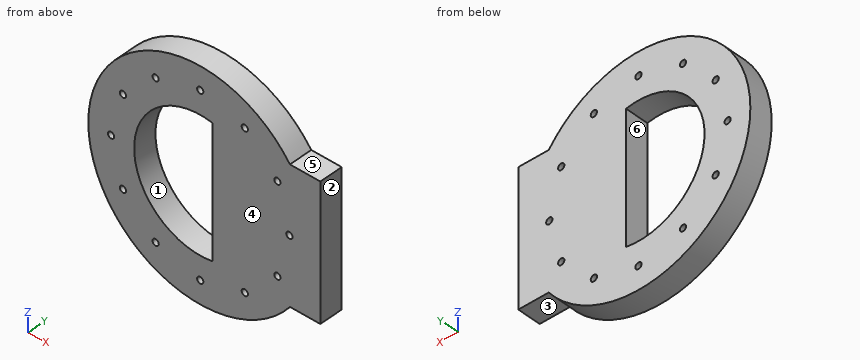
```python
from build123d import *

# Parameters (mm, degrees)
SKETCH1_R           = 127.508
SKETCH1_R_2         = 75.311
SKETCH1_R_3         = 3.5687
BOSS_EXTRUDE1_DEPTH = 26.67
BOSS_EXTRUDE2_DEPTH = 26.67


with BuildPart() as part:
    # Sketch1 → Boss-Extrude1 (new body)
    with BuildSketch(Plane(origin=(0, 0, 0), x_dir=(1, 0, 0), z_dir=(0, 1, 0))):
        Circle(SKETCH1_R)
        Circle(SKETCH1_R_2, mode=Mode.SUBTRACT)
        with Locations((0, 101.6)):
            Circle(SKETCH1_R_3, mode=Mode.SUBTRACT)
        with Locations((50.8, 87.988181024)):
            Circle(SKETCH1_R_3, mode=Mode.SUBTRACT)
        with Locations((87.988181025, 50.8)):
            Circle(SKETCH1_R_3, mode=Mode.SUBTRACT)
        with Locations((101.6, 0)):
            Circle(SKETCH1_R_3, mode=Mode.SUBTRACT)
        with Locations((87.988181025, -50.8)):
            Circle(SKETCH1_R_3, mode=Mode.SUBTRACT)
        with Locations((50.8, -87.988181024)):
            Circle(SKETCH1_R_3, mode=Mode.SUBTRACT)
        with Locations((0, -101.6)):
            Circle(SKETCH1_R_3, mode=Mode.SUBTRACT)
        with Locations((-50.8, -87.988181025)):
            Circle(SKETCH1_R_3, mode=Mode.SUBTRACT)
        with Locations((-87.988181024, -50.8)):
            Circle(SKETCH1_R_3, mode=Mode.SUBTRACT)
        with Locations((-101.6, 0)):
            Circle(SKETCH1_R_3, mode=Mode.SUBTRACT)
        with Locations((-87.988181024, 50.8)):
            Circle(SKETCH1_R_3, mode=Mode.SUBTRACT)
        with Locations((-50.8, 87.988181024)):
            Circle(SKETCH1_R_3, mode=Mode.SUBTRACT)
    extrude(amount=BOSS_EXTRUDE1_DEPTH)

    # Sketch2 → Boss-Extrude2 (add, through all)
    with BuildSketch(Plane(origin=(0, 26.67, 0), x_dir=(1, 0, 0), z_dir=(0, 1, 0))):
        with BuildLine():
            Line((14.224, 73.955557905), (14.224, -73.955557905))
            ThreePointArc((14.224, -73.955557905), (75.311, 0), (14.224, 73.955557905))
        make_face()
        with BuildLine():
            Line((136.906, 76.2), (136.906, -76.2))
            Line((136.906, -76.2), (102.23429006, -76.2))
            ThreePointArc((102.23429006, -76.2), (127.508, 0), (102.23429006, 76.2))
            Line((102.23429006, 76.2), (136.906, 76.2))
        make_face()
    extrude(amount=-BOSS_EXTRUDE2_DEPTH)


solid = part.part
```
Model file for the job. Use its own axes, mm. Face numbers are marked on the shaded views. A direction names the side the tool comes from. Give positions to 0.01 mm unless a question says otherwise; leave off trailing zeros. Loops run counter-clockwise (first coordinate to the right, second up) from the corner with the lowest first, then second, coordinate; pieces in that order, holes last. Notation, with made-up numbers: M 11.25,16.5 L 26.25,16.5 A21 ccw 26.25,29.5 Z; hole C -11,-15 d10. An arc over 180 degrees is marked long. Use one line per item in the form item = value.
Item 1: Two-plate mould, pull along Z, no slides. Class the marked faces 1, 2 and 3: released by +Z, released by -Z, zero draft, split by the parting line, or undercut.
Filled in:
face_1 = undercut
face_2 = zero draft
face_3 = released by -Z
Item 2: Slice it at B-B on z = 68. List the corners of the cut face in (x, y).
Filled in:
outline = M -107.86,0 L -32.37,0 L -32.37,26.67 L -107.86,26.67 Z; M 14.22,0 L 136.91,0 L 136.91,26.67 L 14.22,26.67 Z
Item 3: Slice it at D-D on x = -101.6. List the corners of the cut face in (y, z), and give its area (3 significant figures).
Filled in:
outline = M 0,-77.04 L 26.67,-77.04 L 26.67,-3.57 L 0,-3.57 Z; M 0,3.57 L 26.67,3.57 L 26.67,77.04 L 0,77.04 Z
area = 3,920 mm^2
Item 4: Slice it at C-C on y = 15.5. Give the number of separate pieces and of enclosed holes in the cut face, and give its area (3 significant figures).
Filled in:
separate_pieces = 1
enclosed_holes = 13
area = 42,200 mm^2
Item 5: Drill centre lines: L1, parallel to Z at x = -53.5, y = 4.75; L2, parallel to X at y = 3.5, z = -49.5; L3, parallel to Z at x = 50, y = 23. Where is each one in solid material? Low to high.
Filled in:
L1 = -115.74 to -90.32, -85.65 to -53, 53 to 85.65, 90.32 to 115.74
L2 = -117.51 to -91.31, -84.66 to -56.76, 14.22 to 84.66, 91.31 to 136.91
L3 = -117.3 to -91.47, -84.51 to 84.51, 91.47 to 117.3
Item 6: Which spindle directions (+Z, -Z, +X, -X, +Y, -Y) get a long thin tool onto all of the face, cutting with end or side? Do the marked faces 4, 5 and 6. Say none if no direction does.
Filled in:
face_4 = +Z, -Z, +X, -X, -Y
face_5 = +Z, +X, +Y, -Y
face_6 = +Y, -Y
Item 7: Slice it at A-A on x = 0. List the corners of the cut face in (y, z), and give its area (3 significant figures).
Filled in:
outline = M 0,-127.51 L 26.67,-127.51 L 26.67,-105.17 L 0,-105.17 Z; M 0,-98.03 L 26.67,-98.03 L 26.67,-75.31 L 0,-75.31 Z; M 0,75.31 L 26.67,75.31 L 26.67,98.03 L 0,98.03 Z; M 0,105.17 L 26.67,105.17 L 26.67,127.51 L 0,127.51 Z
area = 2,400 mm^2
Item 8: Flat gauge pins, fed straight in: pin 1 Ø3 at (x, y) = (-19, 9.5) entering from -Z; pin 2 Ø4.5 at (x, z) = (50.8, 87.99) entering from +Y; pin 3 Ø4 at (x, y) = (14.5, 23) entering from -Z; pin 4 Ø8 at (x, y) = (112.5, 10.5) entering from -Z. Where does each tip first touch, or does it go through?
Filled in:
pin_1 = -126.3
pin_2 = through
pin_3 = -126.89
pin_4 = -76.2
